```python
from build123d import *

# Parameters (mm, degrees)
F0_W            = 50
F0_H            = 120
F0_W_2          = 44
F0_H_2          = 44
F1_DEPTH        = 5
F2_W            = 50
F2_H            = 3
F3_DEPTH        = 35
F4_DEPTH        = 15
F5_DEPTH        = 80
F6_W            = 10
F6_H            = 10
F7_W            = 10
F7_H            = 10
F8_DEPTH        = 10
F9_SIZE         = 9.99999
F10_W           = 20
F10_H           = 30
F11_DEPTH       = 3
F12_R           = 6
F13_F1_R        = 2
F13_F2_R        = 2
F13_F3_R        = 2
F13_F4_R        = 2
F13_F5_R        = 2
F13_F6_R        = 2
F13_F7_R        = 2
F13_F8_R        = 2
F13_F9_R        = 2
F13_F10_R       = 2
F13_F11_R       = 2
F13_F12_R       = 2
F13_F13_R       = 2
F13_F14_R       = 2
F13_F15_R       = 2
F13_F16_R       = 2
F13_F17_R       = 2
F13_F18_R       = 2
F13_F19_R       = 2
F13_F20_R       = 2
F15_D           = 4.2
F15_DEPTH       = 12
F15_CSINK_D     = 8.96
F15_CSINK_ANGLE = 90
F15_TIP         = 1.2618073


# Not quite as in the source:
# - a fillet or chamfer is up to 0.001 mm smaller than in the source, because OpenCascade refuses the exact size


with BuildPart() as f1:
    # F0 (on Top) → F1 (new body)
    with BuildSketch(Plane.XY):
        with Locations((0, 11.5)):
            Rectangle(F0_W, F0_H)
        with Locations((0, -23.5)):
            Rectangle(F0_W_2, F0_H_2, mode=Mode.SUBTRACT)
        with Locations((0, 23.5)):
            Rectangle(F0_W_2, F0_H_2, mode=Mode.SUBTRACT)
    extrude(amount=F1_DEPTH)

    # F2 (on face) → F3 (join)
    with BuildSketch(Plane.XY.offset(5)):
        with Locations((0, 70)):
            Rectangle(F2_W, F2_H)
    extrude(amount=F3_DEPTH)

    # F2 (on face) → F4 (join)
    with BuildSketch(Plane.XY.offset(5)):
        Polygon((25, 48.5), (-25, 48.5), (-25, 45.5), (-22, 45.5), (22, 45.5), (25, 45.5), align=None)
    extrude(amount=F4_DEPTH)

    # F2 (on face) → F5 (join)
    with BuildSketch(Plane.XY.offset(5)):
        Polygon((-22, 11.5), (-25, 11.5), (-25, -1.5), (-22, -1.5), (-12, -1.5), (-12, 1.5), (-22, 1.5), align=None)
        Polygon((25, -1.5), (25, 11.5), (22, 11.5), (22, 1.5), (12, 1.5), (12, -1.5), (22, -1.5), align=None)
        Polygon((-22, -35.5), (-25, -35.5), (-25, -48.5), (-12, -48.5), (-12, -45.5), (-22, -45.5), align=None)
        Polygon((25, -48.5), (25, -35.5), (22, -35.5), (22, -45.5), (12, -45.5), (12, -48.5), align=None)
    extrude(amount=F5_DEPTH)

    # F6 (on face) + F7 (on face) → F8 (join)
    with BuildSketch(Plane(origin=(0, 1.5, 0), x_dir=(-1, 0, 0), z_dir=(0, 1, 0))):
        with Locations((-17, 80)):
            Rectangle(F6_W, F6_H)
        with Locations((17, 80)):
            Rectangle(F6_W, F6_H)
    with BuildSketch(Plane(origin=(0, -45.5, 0), x_dir=(-1, 0, 0), z_dir=(0, 1, 0))):
        with Locations((17, 80)):
            Rectangle(F7_W, F7_H)
        with Locations((-17, 80)):
            Rectangle(F7_W, F7_H)
    extrude(amount=F8_DEPTH)

    # F9 (size 10 in the source; OpenCascade refuses exactly that, so slightly less here)
    f9_edges = [f1.edges().sort_by_distance(p)[0] for p in [
        (-17, 11.5, 75),
        (-17, -35.5, 75),
        (17, 11.5, 75),
        (17, -35.5, 75),
    ]]
    chamfer(f9_edges, length=F9_SIZE)

    # F10 (on face) → F11 (cut, through all)
    with BuildSketch(Plane(origin=(0, 71.5, 0), x_dir=(-1, 0, 0), z_dir=(0, 1, 0))):
        with Locations((0, 25)):
            Rectangle(F10_W, F10_H)
    extrude(amount=-F11_DEPTH, mode=Mode.SUBTRACT)

    # F12
    f12_edges = [f1.edges().sort_by_distance(p)[0] for p in [
        (25, 70, 40),
        (10, 70, 40),
        (-10, 70, 40),
        (-25, 70, 40),
    ]]
    fillet(f12_edges, radius=F12_R)

    # F13: fillet of radius 2 on 36 edges, made by hand

    # F13_f1
    f13_f1_edges = [f1.edges().sort_by_distance(p)[0] for p in [
        (25, 71.5, 17),
        (23.2426406871, 71.5, 38.2426406871),
        (17.5, 71.5, 40),
        (11.7573593129, 71.5, 38.2426406871),
        (10, 71.5, 22),
    ]]
    fillet(f13_f1_edges, radius=F13_F1_R)

    # F13_f2
    f13_f2_edges = [f1.edges().sort_by_distance(p)[0] for p in [
        (25, 10.5, 0),
    ]]
    fillet(f13_f2_edges, radius=F13_F2_R)

    # F13_f3
    f13_f3_edges = [f1.edges().sort_by_distance(p)[0] for p in [
        (25, 47, 20),
    ]]
    fillet(f13_f3_edges, radius=F13_F3_R)

    # F13_f4
    f13_f4_edges = [f1.edges().sort_by_distance(p)[0] for p in [
        (25, -48.5, 43.5),
    ]]
    fillet(f13_f4_edges, radius=F13_F4_R)

    # F13_f5
    f13_f5_edges = [f1.edges().sort_by_distance(p)[0] for p in [
        (25, -35.5, 45),
    ]]
    fillet(f13_f5_edges, radius=F13_F5_R)

    # F13_f6
    f13_f6_edges = [f1.edges().sort_by_distance(p)[0] for p in [
        (25, 11.5, 45),
    ]]
    fillet(f13_f6_edges, radius=F13_F6_R)

    # F13_f7
    f13_f7_edges = [f1.edges().sort_by_distance(p)[0] for p in [
        (25, -1.5, 45),
    ]]
    fillet(f13_f7_edges, radius=F13_F7_R)

    # F13_f8
    f13_f8_edges = [f1.edges().sort_by_distance(p)[0] for p in [
        (-25, 71.5, 18),
        (-23.2426406871, 71.5, 38.2426406871),
        (-17.5, 71.5, 40),
        (-11.7573593129, 71.5, 38.2426406871),
        (-10, 71.5, 22),
    ]]
    fillet(f13_f8_edges, radius=F13_F8_R)

    # F13_f9
    f13_f9_edges = [f1.edges().sort_by_distance(p)[0] for p in [
        (-25, -35.5, 45),
    ]]
    fillet(f13_f9_edges, radius=F13_F9_R)

    # F13_f10
    f13_f10_edges = [f1.edges().sort_by_distance(p)[0] for p in [
        (-25, 47, 20),
    ]]
    fillet(f13_f10_edges, radius=F13_F10_R)

    # F13_f11
    f13_f11_edges = [f1.edges().sort_by_distance(p)[0] for p in [
        (-25, -1.5, 45),
    ]]
    fillet(f13_f11_edges, radius=F13_F11_R)

    # F13_f12
    f13_f12_edges = [f1.edges().sort_by_distance(p)[0] for p in [
        (-25, 11.5, 45),
    ]]
    fillet(f13_f12_edges, radius=F13_F12_R)

    # F13_f13
    f13_f13_edges = [f1.edges().sort_by_distance(p)[0] for p in [
        (-22, 45.5, 2.5),
    ]]
    fillet(f13_f13_edges, radius=F13_F13_R)

    # F13_f14
    f13_f14_edges = [f1.edges().sort_by_distance(p)[0] for p in [
        (22, 45.5, 2.5),
    ]]
    fillet(f13_f14_edges, radius=F13_F14_R)

    # F13_f15
    f13_f15_edges = [f1.edges().sort_by_distance(p)[0] for p in [
        (-22, -1.5, 2.5),
    ]]
    fillet(f13_f15_edges, radius=F13_F15_R)

    # F13_f16
    f13_f16_edges = [f1.edges().sort_by_distance(p)[0] for p in [
        (22, -1.5, 2.5),
    ]]
    fillet(f13_f16_edges, radius=F13_F16_R)

    # F13_f17
    f13_f17_edges = [f1.edges().sort_by_distance(p)[0] for p in [
        (-22, -45.5, 37.5),
    ]]
    fillet(f13_f17_edges, radius=F13_F17_R)

    # F13_f18
    f13_f18_edges = [f1.edges().sort_by_distance(p)[0] for p in [
        (22, -45.5, 37.5),
    ]]
    fillet(f13_f18_edges, radius=F13_F18_R)

    # F13_f19
    f13_f19_edges = [f1.edges().sort_by_distance(p)[0] for p in [
        (-22, 1.5, 37.5),
    ]]
    fillet(f13_f19_edges, radius=F13_F19_R)

    # F13_f20
    f13_f20_edges = [f1.edges().sort_by_distance(p)[0] for p in [
        (22, 1.5, 37.5),
    ]]
    fillet(f13_f20_edges, radius=F13_F20_R)

    # F15
    with Locations(Plane(origin=(0, 71.5, 0), x_dir=(-1, 0, 0), z_dir=(0, 1, 0))):
        with Locations((-17.5, 22), (17.5, 22)):
            CounterSinkHole(F15_D / 2, F15_CSINK_D / 2, depth=F15_DEPTH, counter_sink_angle=F15_CSINK_ANGLE)
            with Locations((0, 0, -(F15_DEPTH + F15_TIP / 2))):  # 118° drill point
                Cone(0, F15_D / 2, F15_TIP, mode=Mode.SUBTRACT)


solid = f1.part
```
The model under review builds one solid part; all positions refer to its coordinate system, in mm. A direction names the side the tool comes from. Coordinates: 2 decimals unless noted, no trailing zeros. Write each loop counter-clockwise with the first axis right and the second up, starting at its lowest first coordinate (ties: lowest second). Pieces come first, ordered by that corner, then holes. Notation, with made-up numbers: (76.25, 5) - (108.25, 5) arc R13 ccw to (108.25, 22) - close; hole circle Ø1 at (42.25, 12.25). An arc over 180 degrees is marked (long way). Answer in a Markdown table with one row per item. Add a question column.
Q1. Draft analysis for pull direction Z (two halves, no side actions). For faces 5 (the face through (11.804, 68.993, 38.289)), 6 (the face through (0, 71.5, 8)), 7 (the face through (-15.497, 68.806, 22.631)), state which applies: +Z half, -Z half, draft (parallel to the pull), parting line (faces both ways), or undercut.
Q2. To check wall thickness, follow line 1 along X through (y, z) = (68.9, 22); line 2 along Y through (x, z) = (14, 25.5); line 3 along Z through (x, y) = (17.5, 68.6). State the ranges of each line that lie inside material, in increasing order. Write a range as from..to.
Q3. Consider section D-D on y = 62. Give the boundary of the cut face in (x, z), then the cut area to 3 significant figures.
Q4. For faces 1 (the face through (-22, -37, 30)), 2 (the face through (-22.8, 11.5, 44.8)), 3 (the face through (0, 45.5, 10)), 4 (the face through (-12, 1, 51)), list the 3-axis set-ups (+Z, -Z, +X, -X, +Y, -Y) from which the entire face can be reached by the end or side of a thin tool; tool diameter is ignored.
Q5. Consider section C-C on x = -17.5. Give the number of separate pieces and of enclosed holes in the cut face, then the cut area to 3 significant figures.
Q6. Consider section B-B on y = -14. Give the boundary of the cut face in (x, z), then the cut area to 3 significant figures.
Q7. Consider section A-A on x = -6. Give the boundary of the cut face in (y, z).
Q8. Clearance check with flat-ended pins moving along their axes: pin 1 (0.8 mm diameter, centred on x = 17, y = 69, fed in from +Z); pin 2 (3.5 mm diameter, centred on x = -1.5, y = 0.5, fed in from +Z); pin 3 (3.5 mm diameter, centred on x = 3, y = 70, fed in from +Z). State where each tip first meets the part, or that it passes through.
Answers below:
| question | item | result |
|---|---|---|
| 1 | face 5 | +Z half |
| 1 | face 6 | draft |
| 1 | face 7 | undercut |
| 2 | line 1 | -25..-19.6, -15.4..-10, 10..15.4, 19.6..25 |
| 2 | line 2 | -48.5..-45.5, -1.5..1.5, 68.5..71.5 |
| 2 | line 3 | 0..19.9, 24.1..40 |
| 3 | outline | (-25, 2) arc R2 ccw to (-23, 0) - (23, 0) arc R2 ccw to (25, 2) - (25, 5) - (-25, 5) - close |
| 3 | area | 248 mm² |
| 4 | face 1 | -Z |
| 4 | face 2 | +Z, +X, -X |
| 4 | face 3 | +Z |
| 4 | face 4 | +Z, -Y |
| 5 | separate pieces | 4 |
| 5 | enclosed holes | 0 |
| 5 | area | 869 mm² |
| 6 | outline | (-25, 2) arc R2 ccw to (-23, 0) - (-22, 0) - (-22, 5) - (-25, 5) - close; (22, 0) - (23, 0) arc R2 ccw to (25, 2) - (25, 5) - (22, 5) - close |
| 6 | area | 28.3 mm² |
| 7 | outline | (-48.5, 2) arc R2 ccw to (-46.5, 0) - (-45.5, 0) - (-45.5, 5) - (-48.5, 5) - close; (-1.5, 0) - (1.5, 0) - (1.5, 5) - (-1.5, 5) - close; (45.5, 0) - (69.5, 0) arc R2 ccw to (71.5, 2) - (71.5, 10) - (68.5, 10) - (68.5, 5) - (48.5, 5) - (48.5, 20) - (45.5, 20) - close |
| 8 | pin 1 | z = 40 |
| 8 | pin 2 | z = 5 |
| 8 | pin 3 | z = 10 |
